The drawing under review shows one solid part. Ordinate dimensions are in mm from its lowest x, y, z. A direction names the side the tool comes from. Give positions to 0.01 mm unless a question says otherwise; leave off trailing zeros. Write each loop counter-clockwise with the first axis right and the second up, starting at its lowest first coordinate (ties: lowest second). Pieces come first, ordered by that corner, then holes. Notation, with made-up numbers: M 44,38.25 L 72,38.25 A17 ccw 72,54.25 Z; hole C 32,43.25 d10. An arc over 180 degrees is marked long. Write item = value, one per line. Start each with the question number.
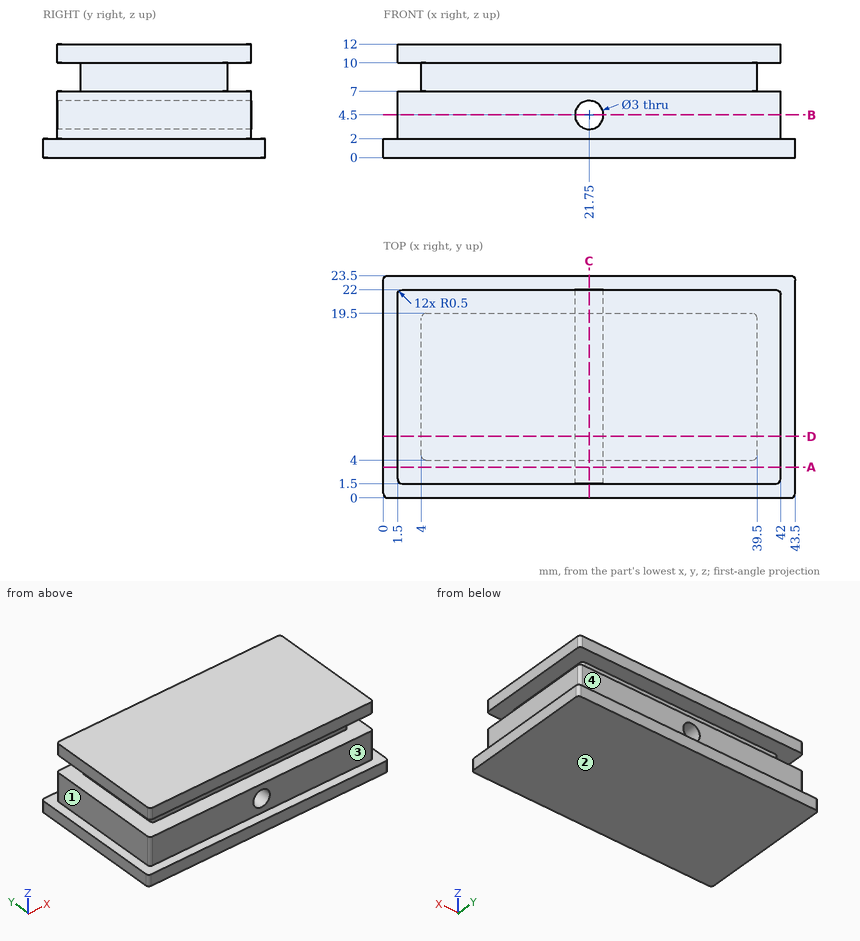
Item 1: For the marked faces 1, 2, 3 and 4, list the 3-axis set-ups (+Z, -Z, +X, -X, +Y, -Y) from which the entire face can be reached by the end or side of a thin tool; tool diameter is ignored.
Item 2: We need section B-B, the plane z = 4.5. Write out the cut boundary in (x, y), and give its area (3 significant figures).
Item 3: We need section D-D, the plane y = 6.5. Write out the cut boundary in (x, z).
Item 4: Clearance check with flat-ended pins moving along their axes: P1, Ø1.6, axis at y = 10.5, z = 11, coming from the -X side; P2, Ø1, axis at x = 27.5, z = 11, coming from the +Y side; P3, Ø2, axis at y = 7, z = 11, coming from the +X side; P4, Ø2, axis at x = 39, z = 2.5, coming from the +Y side. State where each tip first meets the part, or that it passes through.
Item 5: We need section A-A, the plane y = 3.25. Write out the cut boundary in (x, z).
Item 6: We need section C-C, the plane x = 21.75. Write out the cut boundary in (y, z).
Item 7: To check wall thickness, follow probe 1 along Z at (x, y) = (21.75, 9.25); probe 2 along Z at (x, y) = (28, 3.5); probe 3 along Y at (x, z) = (37, 6.25). State the ranges of each line that lie inside material, in increasing order. Write a range as [from, to].
Worked out:
q1.face_1 = +Z, -X, +Y, -Y
q1.face_2 = -Z, +X, -X, +Y, -Y
q1.face_3 = +Z, +X, -X, -Y
q1.face_4 = +Z, +X, -X, +Y
q2.outline = M 1.5,2 A0.5 ccw 2,1.5 L 20.25,1.5 L 20.25,22 L 2,22 A0.5 ccw 1.5,21.5 Z; M 23.25,1.5 L 41.5,1.5 A0.5 ccw 42,2 L 42,21.5 A0.5 ccw 41.5,22 L 23.25,22 Z
q2.area = 769 mm²
q3.outline = M 0,0 L 43.5,0 L 43.5,2 L 42,2 L 42,7 L 39.5,7 L 39.5,10 L 42,10 L 42,12 L 1.5,12 L 1.5,10 L 4,10 L 4,7 L 1.5,7 L 1.5,2 L 0,2 Z; hole C 21.75,4.5 d3
q4.P1 = 1.5
q4.P2 = 22
q4.P3 = 42
q4.P4 = 23.5
q5.outline = M 0,0 L 43.5,0 L 43.5,2 L 42,2 L 42,7 L 1.5,7 L 1.5,2 L 0,2 Z; M 1.5,10 L 42,10 L 42,12 L 1.5,12 Z; hole C 21.75,4.5 d3
q6.outline = M 0,0 L 23.5,0 L 23.5,2 L 22,2 L 22,3 L 1.5,3 L 1.5,2 L 0,2 Z; M 1.5,6 L 22,6 L 22,7 L 19.5,7 L 19.5,10 L 22,10 L 22,12 L 1.5,12 L 1.5,10 L 4,10 L 4,7 L 1.5,7 Z
q7.probe_1 = [0, 3], [6, 12]
q7.probe_2 = [0, 7], [10, 12]
q7.probe_3 = [1.5, 22]
